Could you check a few things on this model? Use its own coordinates, in mm. A direction names the side the tool comes from. Round coordinates to 2 decimals unless told otherwise and drop trailing zeros. Write each loop counter-clockwise with the first axis right and the second up, starting at its lowest first coordinate (ties: lowest second). Pieces come first, ordered by that corner, then holes. Notation, with made-up numbers: (34, -37.75) -> (60, -37.75) arc R19 ccw to (60, -27.75) -> close; hole circle Ø8 at (19.5, -14). An arc over 180 degrees is marked (long way). One line per question, with ' | ' between items. Start each with the question number.
1. Imagine slicing it at C-C, the plane y = 36. List the corners of the cut face in (x, z) for me, and give its area (3 significant figures).
2. Thinking about a two-plate mould opening in Y: for faces 1 (the cylindrical face through (11.054, -12.744, 2.535)), 2 (the cylindrical face through (-6.9, 39.43, -54.74)), 3 (the cylindrical face through (10.12, -7.01, 2.46)), which applies, released by +Y, released by -Y, zero draft, split by the parting line, or undercut?
3. Imagine slicing it at A-A, the plane z = -45. List the corners of the cut face in (x, y) for me.
4. If I drill on line 1 along Z through (x, y) = (5.5, 35.5); line 2 along Z through (x, y) = (10.5, 6); line 3 along Y through (x, z) = (-5.5, -50.5), over which ranges is the centre line in solid material (lowest first)? Write a range as [from, to].
5. Imagine slicing it at B-B, the plane y = -2.5. List the corners of the cut face in (x, z) for me.
6. For faces 4 (the cylindrical face through (13.5, 0.05, 2.46)), 5 (the flat face through (-4, 37.3, -42)), 6 (the flat face through (-7.5, 36, -27)), 7 (the flat face through (4.696, 19.476, 2.535)), which set-ups out of +Z, -Z, +X, -X, +Y, -Y let a thin tool reach every point of the face, with its end or its side?
7. For pin 1 Ø4.5 at (x, z) = (-2.5, -23) entering from -Y; pin 2 Ø1.5 at (y, z) = (13.5, 1.5) entering from -X; pin 3 Ø10 at (y, z) = (34, -13) entering from -X; pin 4 Ø3.5 at (x, z) = (-4.42, -40.58) entering from +Y, each with a flat end and sliding along its axis, tell me the tip position at first contact or that it passes through.
8. Imagine slicing it at D-D, the plane z = -2. List the corners of the cut face in (x, y) for me.
from build123d import *

# Parameters (mm, degrees)
SKETCH_1_R                   = 1
SKETCH_1_R_2                 = 1.25
EXTRUDE_1_DEPTH              = 5
EXTRUDE_2_DEPTH              = 7.5
SKETCH_5_R                   = 2.25
CUT_EXTRUDE_1_DEPTH          = 15
FILLET_2_R                   = 40
HOLE_WIZARD_M2_1_D           = 2.2
HOLE_WIZARD_M2_1_CBORE_D     = 4.3
HOLE_WIZARD_M2_1_CBORE_DEPTH = 2.3
CUT_EXTRUDE_2_DEPTH          = 79.302298817
FILLET_1_R                   = 2


with BuildPart() as part:
    # 草图1 → 凸台-拉伸1 (new body)
    # profile 1 of 2: a face of its own
    with BuildSketch(Plane.XY):
        with BuildLine():
            ThreePointArc((7.5, 15.811388301), (0, 17.5), (-7.5, 15.811388301))
            ThreePointArc((-7.5, 15.811388301), (-17.382056071, 2.028331029), (-10.939015625, -13.659719512))
            Line((-10.939015625, -13.659719512), (-6.250866071, -7.805554007))
            ThreePointArc((-6.250866071, -7.805554007), (-4.329626963, 9.01411839), (10, 0))
            ThreePointArc((10, 0), (9.01411839, -4.329626963), (6.250866071, -7.805554007))
            Line((6.250866071, -7.805554007), (10.939015625, -13.659719512))
            ThreePointArc((10.939015625, -13.659719512), (15.774707183, -7.576847186), (17.5, 0))
            ThreePointArc((17.5, 0), (14.790199458, 9.354143467), (7.5, 15.811388301))
        make_face()
        with Locations((-10.25, -8)):
            Circle(SKETCH_1_R, mode=Mode.SUBTRACT)
        with Locations((-14.75, 0)):
            Circle(SKETCH_1_R_2, mode=Mode.SUBTRACT)
        with Locations((-10.25, 8)):
            Circle(SKETCH_1_R, mode=Mode.SUBTRACT)
        with Locations((10.25, -8)):
            Circle(SKETCH_1_R, mode=Mode.SUBTRACT)
        with Locations((14.75, 0)):
            Circle(SKETCH_1_R_2, mode=Mode.SUBTRACT)
        with Locations((10.25, 8)):
            Circle(SKETCH_1_R, mode=Mode.SUBTRACT)
    # profile 2 of 2: a face of its own
    with BuildSketch(Plane.XY):
        with BuildLine():
            Line((-7.5, 40), (-7.5, 15.811388301))
            ThreePointArc((-7.5, 15.811388301), (0, 17.5), (7.5, 15.811388301))
            Line((7.5, 15.811388301), (7.5, 40))
            Line((7.5, 40), (-7.5, 40))
        make_face()
    extrude(amount=EXTRUDE_1_DEPTH)

    # 草图3 → 凸台-拉伸2 (add, symmetric)
    with BuildSketch(Plane(origin=(0, 0, 0), x_dir=(0, 0, -1), z_dir=(1, 0, 0))):
        Polygon((0, 40), (60, 40), (60, 35), (6, 35), (0, 29), align=None)
    extrude(amount=EXTRUDE_2_DEPTH, both=True)

    # 草图5 → 切除-拉伸1 (cut)
    with BuildSketch(Plane.XZ.offset(-35)):
        with Locations(Location((0, -45, 0), (0, 0, 270))):
            Circle(SKETCH_5_R)
    extrude(amount=-CUT_EXTRUDE_1_DEPTH, mode=Mode.SUBTRACT)

    # 圆角2
    # the kernel refuses this fillet: 40 mm, written as the material it adds along each edge
    with BuildSketch(Plane(origin=(-7.5, 15.811388301, -41.480787978), x_dir=(-0.759976311594863, -0.6499507718394276, 0), z_dir=(0, 0, 1))) as fillet_2_piece_1_section:
        with BuildLine():
            CenterArc((19.614864399, -38.607797373), FILLET_2_R, 105.160956859, 34.301152757)
            Line((-10.784188065, -12.6097665), (0, 0))
            ThreePointArc((0, 0), (4.576801693, -0.609088649), (9.153603386, 0))
        make_face()
    fillet_2_piece_1 = extrude(amount=46.480787978, mode=Mode.PRIVATE)
    fillet_2_piece_1 = split(fillet_2_piece_1, bisect_by=Plane(origin=(-7.11257259, 31.242526898, 0), z_dir=(0, 0, -1)), keep=Keep.TOP, mode=Mode.PRIVATE)
    fillet_2_piece_1 = split(fillet_2_piece_1, bisect_by=Plane(origin=(-7.11257259, 30.681895174, -1.681895174), z_dir=(0, 0.7071067811865467, 0.7071067811865486)), keep=Keep.TOP, mode=Mode.PRIVATE)
    add(fillet_2_piece_1)
    with BuildSketch(Plane(origin=(-7.5, 15.811388301, 0), x_dir=(-0.7599763115948637, -0.6499507718394266, 0), z_dir=(0, 0, 1))) as fillet_2_piece_2_section:
        with BuildLine():
            CenterArc((19.614864399, -38.607797373), FILLET_2_R, 105.160956859, 34.301152757)
            Line((-10.784188065, -12.6097665), (0, 0))
            ThreePointArc((0, 0), (4.576801693, -0.609088649), (9.153603386, 0))
        make_face()
    fillet_2_piece_2 = extrude(amount=5, mode=Mode.PRIVATE)
    fillet_2_piece_2 = split(fillet_2_piece_2, bisect_by=Plane(origin=(-9.04323472, 22.224032405, 6.775967595), z_dir=(0, -0.7071067811865467, -0.7071067811865486)), keep=Keep.TOP, mode=Mode.PRIVATE)
    add(fillet_2_piece_2)
    with BuildSketch(Plane(origin=(-7.5, 15.811388301, 0), x_dir=(-0.7599763115948637, -0.6499507718394266, 0), z_dir=(0, 0, 1))) as fillet_2_piece_3_section:
        with BuildLine():
            CenterArc((19.614864399, -38.607797373), FILLET_2_R, 105.160956859, 34.301152757)
            Line((-10.784188065, -12.6097665), (0, 0))
            ThreePointArc((0, 0), (4.576801693, -0.609088649), (9.153603386, 0))
        make_face()
    fillet_2_piece_3 = extrude(amount=5, mode=Mode.PRIVATE)
    fillet_2_piece_3 = split(fillet_2_piece_3, bisect_by=Plane(origin=(-7.203009065, 27.482958496, 1.517041504), z_dir=(0, 0.7071067811865467, 0.7071067811865486)), keep=Keep.TOP, mode=Mode.PRIVATE)
    add(fillet_2_piece_3)
    with BuildSketch(Plane(origin=(7.5, 15.811388301, -41.480787978), x_dir=(0.7599763115948623, -0.6499507718394282, 0), z_dir=(0, 0, 1))) as fillet_2_piece_4_section:
        with BuildLine():
            CenterArc((19.614864399, 38.607797373), FILLET_2_R, 220.537890384, 34.301152757)
            Line((-10.784188065, 12.6097665), (0, 0))
            ThreePointArc((0, 0), (4.576801693, 0.609088649), (9.153603386, 0))
        make_face()
    fillet_2_piece_4 = extrude(amount=46.480787978, mode=Mode.PRIVATE)
    fillet_2_piece_4 = split(fillet_2_piece_4, bisect_by=Plane(origin=(7.11257259, 31.242526898, 0), z_dir=(0, 0, -1)), keep=Keep.TOP, mode=Mode.PRIVATE)
    fillet_2_piece_4 = split(fillet_2_piece_4, bisect_by=Plane(origin=(7.11257259, 30.681895174, -1.681895174), z_dir=(0, 0.7071067811865467, 0.7071067811865486)), keep=Keep.TOP, mode=Mode.PRIVATE)
    add(fillet_2_piece_4)
    with BuildSketch(Plane(origin=(7.5, 15.811388301, 0), x_dir=(0.7599763115948623, -0.6499507718394282, 0), z_dir=(0, 0, 1))) as fillet_2_piece_5_section:
        with BuildLine():
            CenterArc((19.614864399, 38.607797373), FILLET_2_R, 220.537890384, 34.301152757)
            Line((-10.784188065, 12.6097665), (0, 0))
            ThreePointArc((0, 0), (4.576801693, 0.609088649), (9.153603386, 0))
        make_face()
    fillet_2_piece_5 = extrude(amount=5, mode=Mode.PRIVATE)
    fillet_2_piece_5 = split(fillet_2_piece_5, bisect_by=Plane(origin=(9.04323472, 22.224032405, 6.775967595), z_dir=(0, -0.7071067811865467, -0.7071067811865486)), keep=Keep.TOP, mode=Mode.PRIVATE)
    add(fillet_2_piece_5)
    with BuildSketch(Plane(origin=(7.5, 15.811388301, 0), x_dir=(0.7599763115948623, -0.6499507718394282, 0), z_dir=(0, 0, 1))) as fillet_2_piece_6_section:
        with BuildLine():
            CenterArc((19.614864399, 38.607797373), FILLET_2_R, 220.537890384, 34.301152757)
            Line((-10.784188065, 12.6097665), (0, 0))
            ThreePointArc((0, 0), (4.576801693, 0.609088649), (9.153603386, 0))
        make_face()
    fillet_2_piece_6 = extrude(amount=5, mode=Mode.PRIVATE)
    fillet_2_piece_6 = split(fillet_2_piece_6, bisect_by=Plane(origin=(7.203009065, 27.482958496, 1.517041504), z_dir=(0, 0.7071067811865467, 0.7071067811865486)), keep=Keep.TOP, mode=Mode.PRIVATE)
    add(fillet_2_piece_6)

    # M2 六角圆柱头螺钉的柱形沉头孔1 (through all)
    with Locations(Plane(origin=(0, 35, 0), x_dir=(-1, 0, 0), z_dir=(0, -1, 0))):
        with Locations((4.419417382, 40.580582618), (-4.419417382, 40.580582618), (-4.419417382, 49.419417382), (4.419417382, 49.419417382)):
            CounterBoreHole(HOLE_WIZARD_M2_1_D / 2, HOLE_WIZARD_M2_1_CBORE_D / 2, HOLE_WIZARD_M2_1_CBORE_DEPTH)

    # 草图9 → 切除-拉伸2 (cut, through all)
    with BuildSketch(Plane.XY.offset(5)):
        Polygon((-3, 24), (-6, 16), (-6, 8), (6, 8), (6, 16), (3, 24), align=None)
    extrude(amount=-CUT_EXTRUDE_2_DEPTH, mode=Mode.SUBTRACT)

    # 圆角1
    fillet_1_edges = [part.edges().sort_by_distance(p)[0] for p in [
        (10.939015625, -13.659719512, 2.5),
        (6.250866071, -7.805554007, 2.5),
        (-6.250866071, -7.805554007, 2.5),
        (-10.939015625, -13.659719512, 2.5),
        (-7.5, 40, -27.5),
        (7.5, 40, -27.5),
        (0, 29, 0),
        (0, 35, -6),
        (-7.5, 37.5, -60),
        (7.5, 37.5, -60),
        (-6, 8, 2.5),
        (6, 8, 2.5),
        (6, 16, 2.5),
        (3, 24, 2.5),
        (-6, 16, 2.5),
        (-3, 24, 2.5),
    ]]
    fillet(fillet_1_edges, radius=FILLET_1_R)


solid = part.part
Geometry results:
1) outline: (-7.5, -58) arc R2 ccw to (-5.5, -60) -> (5.5, -60) arc R2 ccw to (7.5, -58) -> (7.5, 5) -> (-7.5, 5) -> close; hole circle Ø4.3 at (-4.42, -49.42); hole circle Ø4.3 at (-4.42, -40.58); hole circle Ø4.5 at (0, -45); hole circle Ø4.3 at (4.42, -49.42); hole circle Ø4.3 at (4.42, -40.58) | area: 899 mm2
2) face 1: released by -Y | face 2: released by +Y | face 3: undercut
3) outline: (-7.5, 35) -> (-2.25, 35) -> (-2.25, 40) -> (-5.5, 40) arc R2 ccw to (-7.5, 38) -> close; (2.25, 35) -> (7.5, 35) -> (7.5, 38) arc R2 ccw to (5.5, 40) -> (2.25, 40) -> close
4) line 1: z = [-60, -51.28], [-47.56, -42.44], [-38.72, 5] | line 2: z = [0, 5] | line 3: y = [37.3, 40]
5) outline: (-17.32, 0) -> (-9.68, 0) -> (-9.68, 5) -> (-17.32, 5) -> close; (9.68, 0) -> (17.32, 0) -> (17.32, 5) -> (9.68, 5) -> close
6) face 4: +Z, -Z | face 5: -Y | face 6: +Z, -Z, -X, +Y | face 7: +Z, -Z, -Y
7) pin 1: stops at y = 35 | pin 2: stops at x = -12.66 | pin 3: stops at x = -7.5 | pin 4: stops at y = 40
8) outline: (-7.52, 31) -> (7.52, 31) arc R40 cw to (7.5, 32.4) -> (7.5, 38) arc R2 ccw to (5.5, 40) -> (-5.5, 40) arc R2 ccw to (-7.5, 38) -> (-7.5, 32.4) arc R40 cw to start
